Verification items for the finished model (mm, model axes). A direction names the side the tool comes from. Give positions to 0.01 mm unless a question says otherwise; leave off trailing zeros. Write each loop counter-clockwise with the first axis right and the second up, starting at its lowest first coordinate (ties: lowest second). Pieces come first, ordered by that corner, then holes. Notation, with made-up numbers: M 84.5,5.5 L 126.5,5.5 A11 cw 126.5,13.5 Z; hole C 32,61 d2. An arc over 180 degrees is marked long. Answer as a JSON object with one key per item and string values.
```python
from build123d import *

# Parameters (mm, degrees)
F0_R     = 50.8
F0_R_2   = 40.64
F1_DEPTH = 7.874


with BuildPart() as f1:
    # F0 (on Top) → F1 (new body)
    with BuildSketch(Plane.XY):
        Circle(F0_R)
        Polygon((2.492998, -45.72), (1.246499, -47.879), (-1.246499, -47.879), (-2.492998, -45.72), (-1.246499, -43.561), (1.246499, -43.561), align=None, mode=Mode.SUBTRACT)
        Circle(F0_R_2, mode=Mode.SUBTRACT)
        Polygon((-42.08768, 22.86), (-40.841181, 25.019), (-38.348182, 25.019), (-37.101683, 22.86), (-38.348182, 20.701), (-40.841181, 20.701), align=None, mode=Mode.SUBTRACT)
        Polygon((37.101683, 22.86), (38.348182, 25.019), (40.841181, 25.019), (42.08768, 22.86), (40.841181, 20.701), (38.348182, 20.701), align=None, mode=Mode.SUBTRACT)
    extrude(amount=F1_DEPTH)


solid = f1.part
```
1) Access from +Z, -Z, +X, -X, +Y, -Y to the whole of each face (thin tool, end or side, straight path). Record for faces 3 (the face through (-4, -41, 0)), 4 (the face through (40, 20.701, 4)).
Completed:
{"face 3": "-Z, +X, -X, +Y, -Y", "face 4": "+Z, -Z"}
2) Section check C-C on x = 26. Record the boundary of the cut face in (y, z), and give its area (3 significant figures).
Completed:
{"outline": "M -43.64,0 L -31.23,0 L -31.23,7.87 L -43.64,7.87 Z; M 31.23,0 L 43.64,0 L 43.64,7.87 L 31.23,7.87 Z", "area": "195 mm2"}
3) Release check for a two-part mould opening along X. For faces 1 (the face through (-4, -41, 7.874)), 2 (the face through (-37.73, 23.95, 3.88)) record: pulls with the +X half, pulls with the -X half, needs draft (parallel to the pull), parting line crosses it, or undercut.
Completed:
{"face 1": "needs draft", "face 2": "undercut"}
4) Go/stop test with flat-tipped pins: pin 1 (2 mm diameter, centred on y = -27.5, z = 4.5, fed in from -X); pin 2 (2.5 mm diameter, centred on x = 0.5, z = 4.5, fed in from -Y); pin 3 (2.5 mm diameter, centred on x = 39.5, z = 3.5, fed in from -Y). Record where each tip stops, or that it passes through.
Completed:
{"pin 1": "stops at x = -43.34", "pin 2": "stops at y = -50.8", "pin 3": "stops at y = -33.43"}
5) Section check B-B on y = 0. Record the boundary of the cut face in (x, z).
Completed:
{"outline": "M -50.8,0 L -40.64,0 L -40.64,7.87 L -50.8,7.87 Z; M 40.64,0 L 50.8,0 L 50.8,7.87 L 40.64,7.87 Z"}
6) Thickness scan on L1, parallel to Y at x = 0, z = 2.5; L2, parallel to X at y = 5.5, z = 4.25; L3, parallel to Y at x = -2, z = 6.5. Record the ranges inside material, lowest first.
Completed:
{"L1": "y = -50.8 to -47.88, -43.56 to -40.64, 40.64 to 50.8", "L2": "x = -50.5 to -40.27, 40.27 to 50.5", "L3": "y = -50.76 to -46.57, -44.87 to -40.59, 40.59 to 50.76"}
7) Section check A-A on x = 0. Record the boundary of the cut face in (y, z).
Completed:
{"outline": "M -50.8,0 L -47.88,0 L -47.88,7.87 L -50.8,7.87 Z; M -43.56,0 L -40.64,0 L -40.64,7.87 L -43.56,7.87 Z; M 40.64,0 L 50.8,0 L 50.8,7.87 L 40.64,7.87 Z"}
